```python
from build123d import *

# Parameters (mm, degrees)
BLOCK_SKETCH_W          = 40
BLOCK_SKETCH_H          = 44
BLOCK_DEPTH             = 22
NECK_SKETCH_W           = 15
NECK_SKETCH_H           = 10.1125
REGULATOR_PORT_SKETCH_W = 15
REGULATOR_PORT_SKETCH_H = 7.2
SIDE_PORT_Y_SKETCH_W    = 5.5
SIDE_PORT_Y_SKETCH_H    = 15
SIDE_PORT_Y_SKETCH_2_W  = 5.5
SIDE_PORT_Y_SKETCH_2_H  = 15
SIDE_PORT_Z_SKETCH_R    = 5.5
SIDE_PORT_Z_DEPTH       = 23
SIDE_START              = -23
SIDE_PORT_Z_SKETCH_2_R  = 5.5
SIDE_PORT_Z_2_DEPTH     = 23


with BuildPart() as part:
    # Block Sketch → Block (new, symmetric)
    with BuildSketch(Plane.XY):
        with Locations((-20, 0)):
            Rectangle(BLOCK_SKETCH_W, BLOCK_SKETCH_H)
    extrude(amount=BLOCK_DEPTH, both=True)

    # Neck Sketch → Neck (revolve)
    with BuildSketch(Plane.XY, mode=Mode.PRIVATE) as neck_sk:
        with Locations((7.5, 5.05625)):
            Rectangle(NECK_SKETCH_W, NECK_SKETCH_H)
    revolve(neck_sk.sketch.rotate(Axis((-1000, 0, 0), (1, 0, 0)), 90), axis=Axis((-1000, 0, 0), (1, 0, 0)))

    # Regulator Port Sketch → Regulator Port (revolve, cut)
    with BuildSketch(Plane.XY, mode=Mode.PRIVATE) as regulator_port_sk:
        with Locations((-33.5, 3.6)):
            Rectangle(REGULATOR_PORT_SKETCH_W, REGULATOR_PORT_SKETCH_H)
    revolve(regulator_port_sk.sketch.rotate(Axis((-1000, 0, 0), (1, 0, 0)), 90), axis=Axis((-1000, 0, 0), (1, 0, 0)), mode=Mode.SUBTRACT)

    # Side Port _Y Sketch → Side Port _Y (revolve, cut)
    with BuildSketch(Plane.XY, mode=Mode.PRIVATE) as side_port_y_sk:
        with Locations((-17.25, 15.5)):
            Rectangle(SIDE_PORT_Y_SKETCH_W, SIDE_PORT_Y_SKETCH_H)
    revolve(side_port_y_sk.sketch.rotate(Axis((-20, -40, 0), (0, 1, 0)), 90), axis=Axis((-20, -40, 0), (0, 1, 0)), mode=Mode.SUBTRACT)

    # Side Port -Y Sketch 2 → Side Port -Y 2 (revolve, cut)
    with BuildSketch(Plane.XY, mode=Mode.PRIVATE) as side_port_y_2_sk:
        with Locations((-17.25, -15.5)):
            Rectangle(SIDE_PORT_Y_SKETCH_2_W, SIDE_PORT_Y_SKETCH_2_H)
    revolve(side_port_y_2_sk.sketch.rotate(Axis((-20, -40, 0), (0, 1, 0)), 90), axis=Axis((-20, -40, 0), (0, 1, 0)), mode=Mode.SUBTRACT)

    # Side Port _Z Sketch → Side Port _Z (cut)
    with BuildSketch(Plane.XY):
        with Locations((-20, 0)):
            Circle(SIDE_PORT_Z_SKETCH_R)
    extrude(amount=SIDE_PORT_Z_DEPTH, mode=Mode.SUBTRACT)

    # Side Port -Z Sketch 2 → Side Port -Z 2 (cut)
    with BuildSketch(Plane.XY.offset(SIDE_START)):
        with Locations((-20, 0)):
            Circle(SIDE_PORT_Z_SKETCH_2_R)
    extrude(amount=SIDE_PORT_Z_2_DEPTH, mode=Mode.SUBTRACT)


solid = part.part
```
Geometry check sheet. Reference: the model listing, model coordinates, mm. A direction names the side the tool comes from. Coordinates: 2 decimals unless noted, no trailing zeros. Loops run counter-clockwise (first coordinate to the right, second up) from the corner with the lowest first, then second, coordinate; pieces in that order, holes last.
Item 1: Sectioned sample at D-D, the plane z = 0. Record the boundary of the cut face in (x, y), then the cut area to 3 significant figures.
Item 2: Sectioned sample at B-B, the plane y = 0. Record the boundary of the cut face in (x, z), then the cut area to 3 significant figures.
Item 3: Sectioned sample at A-A, the plane x = -20. Record the boundary of the cut face in (y, z).
Item 4: Sectioned sample at C-C, the plane x = -27.5. Record the boundary of the cut face in (y, z).
Item 5: Access from +Z, -Z, +X, -X, +Y, -Y to the whole of each face (thin tool, end or side, straight path). Record for faces 1 (the face through (-32.9, -2.16, 6.87)), 2 (the face through (-25.453, 15.098, 0.716)), 3 (the face through (7.6, 8.97, 4.67)).
Item 6: Go/stop test with flat-tipped pins: pin 1 Ø3.5 at (x, z) = (-22.5, 0.5) entering from +Y; pin 2 Ø4.5 at (y, z) = (0, -2.5) entering from -X; pin 3 Ø1.5 at (y, z) = (-10.5, -16) entering from +X; pin 4 Ø6.5 at (x, y) = (-20, 0) entering from -Z. Record where each tip stops, or that it passes through.
Item 7: Release check for a two-part mould opening along Y. For faces 4 (the face through (-26, 0, 0)), 5 (the face through (-25, -22, 5)), 6 (the face through (-25.453, -14.902, 0.716)) record: released by +Y, released by -Y, zero draft, split by the parting line, or undercut.
Item 8: Thickness scan on line 1 (Y direction, x = -20, z = -7); line 2 (X direction, y = 0, z = 0). Record the ranges inside material, lowest first.
Check result:
1. outline: (-40, -22) - (-25.5, -22) - (-25.5, -8) - (-14.5, -8) - (-14.5, -22) - (0, -22) - (0, -10.11) - (15, -10.11) - (15, 10.11) - (0, 10.11) - (0, 22) - (-14.5, 22) - (-14.5, 8) - (-25.5, 8) - (-25.5, 22) - (-40, 22) - (-40, 7.2) - (-26, 7.2) - (-26, -7.2) - (-40, -7.2) - close; hole circle Ø11 at (-20, 0)
1. area: 1,460 mm2
2. outline: (-40, -22) - (-25.5, -22) - (-25.5, 22) - (-40, 22) - (-40, 7.2) - (-26, 7.2) - (-26, -7.2) - (-40, -7.2) - close; (-14.5, -22) - (0, -22) - (0, -10.11) - (15, -10.11) - (15, 10.11) - (0, 10.11) - (0, 22) - (-14.5, 22) - close
2. area: 1,380 mm2
3. outline: (-22, -22) - (-5.5, -22) - (-5.5, 22) - (-22, 22) - (-22, 5.5) - (-8, 5.5) - (-8, -5.5) - (-22, -5.5) - close; (5.5, -22) - (22, -22) - (22, -5.5) - (8, -5.5) - (8, 5.5) - (22, 5.5) - (22, 22) - (5.5, 22) - close
4. outline: (-22, -22) - (22, -22) - (22, 22) - (-22, 22) - close; hole circle Ø14.4 at (0, 0)
5. face 1: -X
5. face 2: +Y
5. face 3: +X
6. pin 1: stops at y = 8
6. pin 2: stops at x = -26
6. pin 3: stops at x = 0
6. pin 4: passes through
7. face 4: undercut
7. face 5: released by -Y
7. face 6: zero draft
8. line 1: y = -22 to -5.5, 5.5 to 22
8. line 2: x = -26 to -25.5, -14.5 to 15
